from build123d import *

# Parameters (mm, degrees)
SKETCH_1_W      = 12.5
SKETCH_1_H      = 5.8
EXTRUDE_1_DEPTH = 6.5
EXTRUDE_2_DEPTH = 5.8


with BuildPart() as part:
    # 草图1 → 凸台-拉伸1 (new body)
    with BuildSketch(Plane(origin=(0, 0, 0), x_dir=(1, 0, 0), z_dir=(0, 1, 0))):
        with Locations((-0.217181467, -0.076640927)):
            Rectangle(SKETCH_1_W, SKETCH_1_H)
    extrude(amount=EXTRUDE_1_DEPTH)

    # 草图2 → 凸台-拉伸2 (add, through all)
    with BuildSketch(Plane.XY.offset(2.976640927)):
        Polygon((6.032818533, 6.5), (-17.62035358, 17.294788047), (-17.703390412, 17.112840569), (5.551104582, 6.5), align=None)
    extrude(amount=-EXTRUDE_2_DEPTH)


solid = part.part
Here's how the part is built. I have some questions about the finished solid (model axes, mm). A direction names the side the tool comes from. Coordinates: 2 decimals unless noted, no trailing zeros. Order: outer loops, then holes, each group sorted by start corner. A loop starts at its lowest first (then second) coordinate and runs counter-clockwise, first axis right, second up.
Item 1: If we mould it in two halves opening along Y, with no side actions, what happens to faces 1 (the face through (-1, 6.5, 0)), 2 (the face through (-5.628, 11.822, 0.117)), 3 (the face through (6.033, 3, 0))? For each: +Y half, -Y half, draft (parallel to the pull), parting line (faces both ways), or undercut.
Result sheet:
face 1: undercut
face 2: +Y half
face 3: draft
Item 2: I need wall thicknesses on line 1 (X direction, y = 3, z = 0.85); line 2 (Y direction, x = 1, z = 1.9); line 3 (Y direction, x = -3.75, z = -1.4). Which ranges of each line are inside material? Lowest first, please.
Result sheet:
line 1: x = -6.47 to 6.03
line 2: y = 0 to 6.5, 8.58 to 8.8
line 3: y = 0 to 6.5, 10.74 to 10.96
Item 3: For faces 4 (the face through (-1, 4, 2.977)), 5 (the face through (-6.467, 3, 0)), 6 (the face through (-6.24, 11.88, 0.12)), which set-ups out of +Z, -Z, +X, -X, +Y, -Y let a thin tool reach every point of the face, with its end or its side?
Result sheet:
face 4: +Z, +X, -X, +Y, -Y
face 5: +Z, -Z, -X, -Y
face 6: +Z, -Z, -X
Item 4: For P1, Ø1.5, axis at y = 7.5, z = -1.5, coming from the +X side (3 decimals); P2, Ø1.7, axis at x = 2.5, z = 0.5, coming from the +Y side; P3, Ø3, axis at x = -13, z = 2, coming from the -Y side, each with a flat end and sliding along its axis, tell me the tip position at first contact or that it passes through.
Result sheet:
P1: stops at x = 5.485
P2: stops at y = 8.5
P3: stops at y = 14.28
Item 5: If we section it at A-A on x = -5.25: List the corners of the cut face in (y, z) for me.
Result sheet:
outline: (0, -2.82) - (6.5, -2.82) - (6.5, 2.98) - (0, 2.98) - close; (11.43, -2.82) - (11.65, -2.82) - (11.65, 2.98) - (11.43, 2.98) - close
Item 6: If we section it at C-C on y = 9.5: List the corners of the cut face in (x, z) for me, plus the area to 3 significant figures.
Result sheet:
outline: (-1.02, -2.82) - (-0.54, -2.82) - (-0.54, 2.98) - (-1.02, 2.98) - close
area: 2.79 mm2
Item 7: If we section it at D-D on x = -15: List the corners of the cut face in (y, z) for me, plus the area to 3 significant figures.
Result sheet:
outline: (15.88, -2.82) - (16.1, -2.82) - (16.1, 2.98) - (15.88, 2.98) - close
area: 1.28 mm2
Item 8: If we section it at B-B on z = -0.75: List the corners of the cut face in (x, y) for me.
Result sheet:
outline: (-17.7, 17.11) - (5.55, 6.5) - (-6.47, 6.5) - (-6.47, 0) - (6.03, 0) - (6.03, 6.5) - (-17.62, 17.29) - close
